from build123d import *

# Parameters (mm, degrees)
SKETCH_W     = 30
SKETCH_H     = 30
PAD_DEPTH    = 2
PAD001_DEPTH = 1


with BuildPart() as part:
    # Sketch → Pad (new body)
    with BuildSketch(Plane.XY):
        Rectangle(SKETCH_W, SKETCH_H)
    extrude(amount=PAD_DEPTH)

    # Sketch001 → Revolution (revolve)
    with BuildSketch(Plane.XZ):
        with BuildLine():
            Line((0, 2), (10, 2))
            Line((10, 2), (10, 4))
            Line((10, 4), (3, 4))
            Line((3, 4), (3, 12.460608))
            ThreePointArc((3, 12.460608), (8.062258, 16.08392), (10, 22))
            Line((8, 22), (10, 22))
            ThreePointArc((0, 14), (5.656854, 16.343146), (8, 22))
            Line((0, 2), (0, 14))
        make_face()
    revolve(axis=Axis((0, 0, 0), (0, 0, 1)))

    # Sketch002 → Pad001 (join, symmetric)
    with BuildSketch(Plane.XZ):
        with BuildLine():
            ThreePointArc((7.544119, 18), (11.285683, 18.617448), (13, 22))
            Line((9, 22), (13, 22))
            Line((7.544119, 18), (9, 22))
        make_face()
    pad001 = extrude(amount=PAD001_DEPTH, both=True)

    # Mirrored: Pad001 across Sketch002 V_Axis
    add(pad001.mirror(Plane(origin=(0, 0, 0), x_dir=(0, -1, 0), z_dir=(1, 0, 0))))


solid = part.part
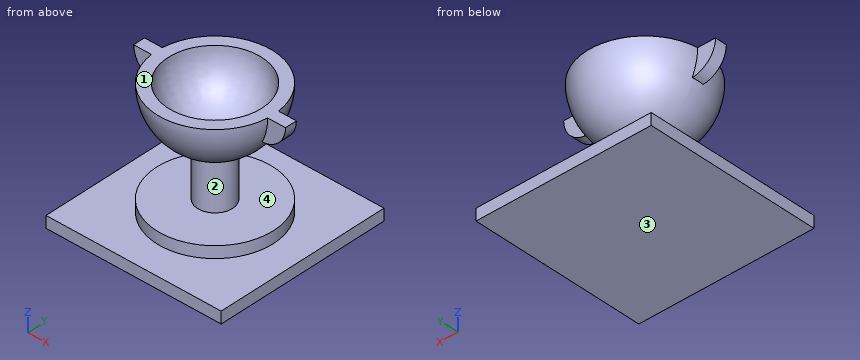
Can you work these out from the model? Positions are in its coordinate system, mm. Face numbers are marked on the shaded views. Coordinates: 2 decimals unless noted, no trailing zeros. Loops run counter-clockwise (first coordinate to the right, second up) from the corner with the lowest first, then second, coordinate; pieces in that order, holes last. Notation, with made-up numbers: M 52,35.25 L 94,35.25 A27 cw 94,70.25 Z; hole C 42,74.5 d3. An arc over 180 degrees is marked long. Return JSON: item names as keys, results as strings. Group by question number.
Item 1: I'm going to push flat-ended pins straight in: pin 1 Ø2 at (y, z) = (9, 2.5) entering from +X; pin 2 Ø1.2 at (x, z) = (11.5, 20) entering from -Y; pin 3 Ø12 at (x, z) = (-3, 19) entering from +Y; pin 4 Ø12 at (y, z) = (5.5, 12.5) entering from -X. Where does each tip first touch, or does it pass through?
Item 2: Imagine slicing it at A-A (z = 10.75). Please give me the cut outline in (x, y).
Item 3: If I drill on L1, parallel to Z at x = -9.75, y = -11.25; L2, parallel to Z at x = -3.25, y = -2; L3, parallel to Y at x = 6.75, z = 19.25, over which ranges is the centre line in solid material (lowest first)? Write a range as from..to.
Item 4: Thinking about a two-plate mould opening in Z: for the marked faces 1, 2, 3 and 4, which applies, released by +Z, released by -Z, zero draft, split by the parting line, or undercut?
Verdict:
{
 "1": {"pin 1": "stops at x = 15", "pin 2": "stops at y = -1", "pin 3": "stops at y = 10", "pin 4": "stops at x = -8.67"},
 "2": {"outline": "C 0,0 d6"},
 "3": {"L1": "z = 0..2", "L2": "z = 0..4, 12.76..14.97", "L3": "y = -6.85..-3.3, 3.3..6.85"},
 "4": {"face 1": "released by +Z", "face 2": "undercut", "face 3": "released by -Z", "face 4": "undercut"}
}
